```python
from build123d import *

# Parameters (mm, degrees)
CYLINDER397_R     = 2
CYLINDER397_DEPTH = 13
CYLINDER396_R     = 2
CYLINDER396_DEPTH = 13
BOX478_W          = 4
BOX478_H          = 4
BOX478_DEPTH      = 4
BOX486_W          = 25
BOX486_H          = 18
BOX486_DEPTH      = 1.5
BOX483_W          = 4
BOX483_H          = 4
BOX483_DEPTH      = 4
BOX485_W          = 4
BOX485_H          = 4
BOX485_DEPTH      = 4
BOX484_W          = 4
BOX484_H          = 4
BOX484_DEPTH      = 4
BOX504_W          = 8
BOX504_H          = 11
BOX504_DEPTH      = 4
BOX505_W          = 8
BOX505_H          = 11
BOX505_DEPTH      = 4


with BuildPart() as cylinder397:
    # Cylinder397 → Cylinder397 (new body)
    with BuildSketch(Plane(origin=(-48, -69, -5), x_dir=(1, 0, 0), z_dir=(0, 0, 1))):
        Circle(CYLINDER397_R)
    extrude(amount=CYLINDER397_DEPTH)


with BuildPart() as fusion394:
    # Cylinder396 → Cylinder396 (new body)
    with BuildSketch(Plane(origin=(-16, -69, -5), x_dir=(1, 0, 0), z_dir=(0, 0, 1))):
        Circle(CYLINDER396_R)
    extrude(amount=CYLINDER396_DEPTH)

    # Fusion394: union Cylinder397
    add(cylinder397.part)


with BuildPart() as fusion394_1:
    # Fusion394 placement: moved
    add(fusion394.part.moved(Location((-2.5, 50, 51))))


with BuildPart() as box478:
    # Box478 → Box478 (new body)
    with BuildSketch(Plane(origin=(-26, -10.5, 51), x_dir=(1, 0, 0), z_dir=(0, 0, 1))):
        with Locations((2, 2)):
            Rectangle(BOX478_W, BOX478_H)
    extrude(amount=BOX478_DEPTH)


with BuildPart() as box486:
    # Box486 → Box486 (new body)
    with BuildSketch(Plane(origin=(-47, -24.5, 53.5), x_dir=(1, 0, 0), z_dir=(0, 0, 1))):
        with Locations((12.5, 9)):
            Rectangle(BOX486_W, BOX486_H)
    extrude(amount=BOX486_DEPTH)


with BuildPart() as box483:
    # Box483 → Box483 (new body)
    with BuildSketch(Plane(origin=(-26, -23.5, 51), x_dir=(1, 0, 0), z_dir=(0, 0, 1))):
        with Locations((2, 2)):
            Rectangle(BOX483_W, BOX483_H)
    extrude(amount=BOX483_DEPTH)


with BuildPart() as box485:
    # Box485 → Box485 (new body)
    with BuildSketch(Plane(origin=(-47, -23.5, 51), x_dir=(1, 0, 0), z_dir=(0, 0, 1))):
        with Locations((2, 2)):
            Rectangle(BOX485_W, BOX485_H)
    extrude(amount=BOX485_DEPTH)


with BuildPart() as box484:
    # Box484 → Box484 (new body)
    with BuildSketch(Plane(origin=(-47, -10.5, 51), x_dir=(1, 0, 0), z_dir=(0, 0, 1))):
        with Locations((2, 2)):
            Rectangle(BOX484_W, BOX484_H)
    extrude(amount=BOX484_DEPTH)


with BuildPart() as box504:
    # Box504 → Box504 (new body)
    with BuildSketch(Plane(origin=(-55, -24.5, 51), x_dir=(1, 0, 0), z_dir=(0, 0, 1))):
        with Locations((4, 5.5)):
            Rectangle(BOX504_W, BOX504_H)
    extrude(amount=BOX504_DEPTH)


with BuildPart() as cut425:
    # Box505 → Box505 (new body)
    with BuildSketch(Plane(origin=(-22, -24.5, 51), x_dir=(1, 0, 0), z_dir=(0, 0, 1))):
        with Locations((4, 5.5)):
            Rectangle(BOX505_W, BOX505_H)
    extrude(amount=BOX505_DEPTH)

    # Fusion395: union Box478, Box486, Box483, Box485, Box484, Box504
    add(box478.part)
    add(box486.part)
    add(box483.part)
    add(box485.part)
    add(box484.part)
    add(box504.part)

    # Cut425: cut Fusion394
    add(fusion394_1.part, mode=Mode.SUBTRACT)


solid = cut425.part
```
Design review of the part built by this model. Coordinates are the model's own, in mm. A direction names the side the tool comes from. Coordinates: 2 decimals unless noted, no trailing zeros. Order: outer loops, then holes, each group sorted by start corner. A loop starts at its lowest first (then second) coordinate and runs counter-clockwise, first axis right, second up. Notation, with made-up numbers: (38.5, -8.5) - (72.5, -8.5) arc R21 cw to (72.5, 0.5) - close; hole circle Ø7 at (46.25, -18). An arc over 180 degrees is marked (long way). Answer in a Markdown table with one row per item.
(1) Consider section B-B on y = -19. State the section outline as (x, z) points, plus the area to 3 significant figures.
Checked values:
| item | result |
|---|---|
| outline | (-55, 51) - (-52.5, 51) - (-52.5, 55) - (-55, 55) - close; (-48.5, 51) - (-47, 51) - (-47, 53.5) - (-22, 53.5) - (-22, 51) - (-20.5, 51) - (-20.5, 55) - (-48.5, 55) - close; (-16.5, 51) - (-14, 51) - (-14, 55) - (-16.5, 55) - close |
| area | 69.5 mm^2 |
(2) Wall thickness on line 1 along X through (y, z) = (-19, 52.4); line 2 along X through (y, z) = (-19, 53.65); line 3 along X through (y, z) = (-23, 51.4): over which ranges is each line inside the solid? List them lowest first. Write a range as from..to.
Checked values:
| item | result |
|---|---|
| line 1 | -55..-52.5, -48.5..-47, -22..-20.5, -16.5..-14 |
| line 2 | -55..-52.5, -48.5..-20.5, -16.5..-14 |
| line 3 | -55..-43, -26..-14 |
(3) For faces 1 (the flat face through (-47, -9, 53)), 2 (the flat face through (-45, -19.5, 52)), 3 (the flat face through (-24, -10.5, 52)), 4 (the flat face through (-26, -9, 52)), 5 (the flat face through (-22, -24, 52)), list the 3-axis set-ups (+Z, -Z, +X, -X, +Y, -Y) from which the entire face can be reached by the end or side of a thin tool; tool diameter is ignored.
Checked values:
| item | result |
|---|---|
| face 1 | +Z, -Z, -X, +Y |
| face 2 | -Z |
| face 3 | -Z, +X, -X |
| face 4 | -Z, +Y, -Y |
| face 5 | -Z, -Y |
(4) Consider section A-A on z = 51.8. State the section outline as (x, y) points, plus the area to 3 significant figures.
Checked values:
| item | result |
|---|---|
| outline | (-55, -24.5) - (-47, -24.5) - (-47, -23.5) - (-43, -23.5) - (-43, -19.5) - (-47, -19.5) - (-47, -13.5) - (-55, -13.5) - close; (-47, -10.5) - (-43, -10.5) - (-43, -6.5) - (-47, -6.5) - close; (-26, -23.5) - (-22, -23.5) - (-22, -24.5) - (-14, -24.5) - (-14, -13.5) - (-22, -13.5) - (-22, -19.5) - (-26, -19.5) - close; (-26, -10.5) - (-22, -10.5) - (-22, -6.5) - (-26, -6.5) - close; hole circle Ø4 at (-50.5, -19); hole circle Ø4 at (-18.5, -19) |
| area | 215 mm^2 |
(5) The part is to be moulded in two halves that separate along X. For faces 6 (the flat face through (-35, -15, 53.5)), 7 (the flat face through (-22, -9, 53)), 8 (the flat face through (-24, -8, 51)), say which applies: released by +X, released by -X, zero draft, split by the parting line, or undercut.
Checked values:
| item | result |
|---|---|
| face 6 | undercut |
| face 7 | released by +X |
| face 8 | zero draft |
(6) Clearance check with flat-ended pins moving along their axes: pin 1 (2 mm diameter, centred on x = -19, z = 53, fed in from +Y); pin 2 (2 mm diameter, centred on x = -24.5, z = 52, fed in from -Y); pin 3 (2 mm diameter, centred on y = -11.5, z = 53.5, fed in from -X). State where each tip first meets the part, or that it passes through.
Checked values:
| item | result |
|---|---|
| pin 1 | y = -13.5 |
| pin 2 | y = -23.5 |
| pin 3 | x = -47 |
(7) Consider section D-D on y = -12.5. State the section outline as (x, z) points, plus the area to 3 significant figures.
Checked values:
| item | result |
|---|---|
| outline | (-47, 53.5) - (-22, 53.5) - (-22, 55) - (-47, 55) - close |
| area | 37.5 mm^2 |
(8) Consider section C-C on x = -18.5. State the section outline as (y, z) points.
Checked values:
| item | result |
|---|---|
| outline | (-24.5, 51) - (-21, 51) - (-21, 55) - (-24.5, 55) - close; (-17, 51) - (-13.5, 51) - (-13.5, 55) - (-17, 55) - close |
